Check sheet for the modelled part. Datum: model origin and axes. Units: mm. A direction names the side the tool comes from. Give positions to 0.01 mm unless a question says otherwise; leave off trailing zeros. Order: outer loops, then holes, each group sorted by start corner. A loop starts at its lowest first (then second) coordinate and runs counter-clockwise, first axis right, second up.
Autodesk Fusion 360 part; units mm, degrees
sketch "Sketch1" plane through (0, 0, 0) normal (0, 1, 0) x (1, 0, 0)
  circle A0 centre (0, 0) radius 42
  dimension "d1" = 84
extrude "Extrude1" add sketch "Sketch1" along normal blind 13
sketch "Sketch2" plane through (0, 13, 0) normal (0, 1, 0) x (-1, 0, 0)
  circle A0 centre (0, 0) radius 42
sketch "Sketch3" plane through (0, 13, 0) normal (0, 1, 0) x (-1, 0, 0)
  line L0 (0, 0) -> (25, 0) construction
  line L1 (0, 0) -> (-25, 0) construction
  line L2 (-25, 0) -> (-25, 11) construction
  line L3 (-25, 11) -> (-25, -10) construction
  line L4 (-25, -10) -> (-40.3348, -10)
  line L5 (-25, 10) -> (-40.5961, 10)
  arc A0 (-25, -10) -> (-25, 10) centre (-25, 0) ccw
  line L6 (-25, -7) -> (-42.662, -7)
  arc A1 (-25, -7) -> (-25, 7) centre (-25, 0) ccw
  line L7 (-25, 7) -> (-45, 7)
  line L8 (-40.3348, -10) -> (-41.543, -10)
  line L9 (-41.543, -10) -> (-46, -10)
  line L10 (-46, -10) -> (-49, 1)
  line L11 (-49, 1) -> (-46.5662, 10.0079)
  line L12 (-46.5662, 10.0079) -> (-40.5961, 10)
  line L13 (-42.662, -7) -> (-45, 7)
  line L14 (0, -45) -> (0, 45) construction
  arc A2 (25, 10) -> (25, -10) centre (25, 0) ccw
  arc A3 (25, 7) -> (25, -7) centre (25, 0) ccw
  line L15 (25, 7) -> (45, 7)
  line L16 (25, 10) -> (40.5961, 10)
  line L17 (46.5662, 10.0079) -> (40.5961, 10)
  line L18 (49, 1) -> (46.5662, 10.0079)
  line L19 (46, -10) -> (49, 1)
  line L20 (25, -10) -> (40.3348, -10)
  line L21 (41.543, -10) -> (46, -10)
  line L22 (42.662, -7) -> (45, 7)
  line L23 (25, -7) -> (42.662, -7)
  line L24 (40.3348, -10) -> (41.543, -10)
  circle A4 centre (0, 0) radius 21
  circle A5 centre (0, 0) radius 11
  circle A6 centre (0, 0) radius 5
  dimension "d4" = 25
  dimension "d5" = 25
  dimension "d7" = 20
  dimension "d8" = 14
  dimension "d13" = 42
  dimension "d14" = 22
  dimension "d15" = 10
extrude "Extrude4" cut sketch "Sketch3" against normal blind 4 contours L4 L5 A0 L6 A1 L7 L8 L9 L10 L11 L12 L13 A4 | A0 A1 A4 | A2 A3 L15 L16 L17 L18 L19 L20 L21 L22 L23 L24 A4 | A2 A3 A4
extrude "Extrude5" cut sketch "Sketch3" against normal blind 13 contours A1 A4 | L6 A1 L7 L13 A4 | A3 L15 L22 L23 A4 | A3 A4
extrude "Extrude6" cut sketch "Sketch3" against normal blind 13 contours A6
extrude "Extrude7" add sketch "Sketch3" along normal blind 6 contours A5
extrude "Extrude8" add sketch "Sketch3" along normal blind 18 contours A0 A2 A4
(1) Cross-section at D-D on y = 27.5. Enter the section's corners in (x, z), then the cut area to 3 significant figures.
Response values:
outline: (-19.32, -8.23) arc R21 ccw to (19.32, -8.23) arc R10 cw to (19.32, 8.23) arc R21 ccw to (-19.32, 8.23) arc R10 cw to start; hole circle Ø22 at (0, 0)
area: 868 mm2
(2) Cross-section at B-B on x = 0. Enter the section's corners in (y, z).
Response values:
outline: (0, -42) - (13, -42) - (13, -21) - (31, -21) - (31, -11) - (19, -11) - (19, -5) - (0, -5) - close; (0, 5) - (19, 5) - (19, 11) - (31, 11) - (31, 21) - (13, 21) - (13, 42) - (0, 42) - close
(3) Material ranges on L1, parallel to Z at x = 0, y = 22.25; L2, parallel to Z at x = 0, y = 8.5; L3, parallel to Y at x = -23.5, z = -16, recorded low to high.
Response values:
L1: z = -21 to -11, 11 to 21
L2: z = -42 to -5, 5 to 42
L3: y = 0 to 13
(4) Cross-section at C-C on x = 9. Enter the section's corners in (y, z), then the cut area to 3 significant figures.
Response values:
outline: (0, -41.02) - (13, -41.02) - (13, -18.97) - (31, -18.97) - (31, -6.32) - (19, -6.32) - (19, 6.32) - (31, 6.32) - (31, 18.97) - (13, 18.97) - (13, 41.02) - (0, 41.02) - close
area: 1,600 mm2
(5) Gauge pin test, flat ends, axial feed: pin 1 Ø1.2 at (x, y) = (-30, 11.5) entering from -Z; pin 2 Ø2 at (x, y) = (33.5, 10.5) entering from +Z; pin 3 Ø4 at (x, y) = (12, 21.5) entering from +Z; pin 4 Ø10 at (x, y) = (-26, 27) entering from +Z. Record the tip position at first contact, or that the pin passes through.
Response values:
pin 1: stops at z = -29.99
pin 2: stops at z = 26.6
pin 3: stops at z = 18.47
pin 4: passes through
(6) Release check for a two-part mould opening along X. For faces 1 (the face through (33, 5, 7)), 2 (the face through (-0.83, 6.41, -41.99)), 3 (the face through (-2, 19, -5)) record: released by +X, released by -X, zero draft, split by the parting line, or undercut.
Response values:
face 1: zero draft
face 2: split by the parting line
face 3: undercut
(7) Set-up check for faces 4 (the face through (-1, 13, -25)), 5 (the face through (-33, 5, -7)), 6 (the face through (-33, 11, -10)), 7 (the face through (2.38, 24.92, 10.74)): record each of +Z, -Z, +X, -X, +Y, -Y from which the full face is reachable in a straight line by a thin tool's end or side.
Response values:
face 4: -Z, +Y
face 5: -X, +Y, -Y
face 6: -X, +Y
face 7: +Y
(8) Cross-section at A-A on y = 7. Enter the section's corners in (x, z).
Response values:
outline: (-41.41, -7) arc R42 ccw to (41.41, -7) - (25, -7) arc R7 cw to (25, 7) - (41.41, 7) arc R42 ccw to (-41.41, 7) - (-25, 7) arc R7 cw to (-25, -7) - close; hole circle Ø10 at (0, 0)
